Autodesk Inventor part; units mm, degrees
ref_plane "YZ Plane" through (0, 0, 0) normal (1, 0, 0) x (0, 1, 0)
ref_plane "XZ Plane" through (0, 0, 0) normal (0, 1, 0) x (-1, 0, 0)
ref_plane "XY Plane" through (0, 0, 0) normal (0, 0, 1) x (1, 0, 0)
sketch "Sketch1" plane through (0, 0, 0) normal (0, 0, 1) x (1, 0, 0)
  line L0 (0, 0) -> (50.8, 0)
  line L1 (50.8, 0) -> (50.8, 25.4)
  line L2 (50.8, 25.4) -> (0, 25.4)
  line L3 (0, 25.4) -> (0, 0)
  line L4 (3.175, 22.225) -> (47.625, 22.225)
  line L5 (47.625, 22.225) -> (47.625, 3.175)
  line L6 (47.625, 3.175) -> (3.175, 3.175)
  line L7 (3.175, 3.175) -> (3.175, 22.225)
  dimension "d0" = 50.8
  dimension "d1" = 25.4
  dimension "d2" = 3.175
extrude "Extrusion1" add sketch "Sketch1" along normal blind 254
sketch "Sketch2" plane through (0, 0, 0) normal (0, -1, 0) x (1, 0, 0)
  circle A0 centre (25.4, 228.6) radius 4.7625
  line L0 (47.625, 254) -> (3.175, 254)
  line L1 (0, 0) -> (0, 254)
  dimension "d5" = 9.525
  dimension "d6" = 25.4
  dimension "d7" = 25.4
extrude "Extrusion2" cut sketch "Sketch2" against normal blind 25.4
sketch "Sketch3" plane through (0, 25.4, 0) normal (0, 1, 0) x (1, 0, 0)
  circle A0 centre (25.4, -228.6) radius 4.7625
  circle A1 centre (25.4, -228.6) radius 14.2875
  point P0 (0, 0)
  dimension "d10" = 28.575
extrude "Extrusion3" cut sketch "Sketch3" against normal blind 25.4
ref_plane "Work Plane1" through (25.4, 0, 228.6) normal (0, 0, -1) x (1, 0, 0)
sketch "Sketch5" plane through (50.8, 0, 0) normal (1, 0, 0) x (0, 0, -1)
  line L0 (-254, 0) -> (-254, 25.4)
  line L1 (0, 0) -> (-254, 0)
  line L2 (0, 25.4) -> (-254, 25.4)
  point P0 (-215.9, 12.7)
  point P1 (-190.5, 12.7)
  point P2 (-165.1, 12.7)
  point P3 (-241.3, 12.7)
  point P4 (-139.7, 12.7)
  dimension "d21" = 38.1
  dimension "d22" = 12.7
  dimension "d23" = 25.4
  dimension "d24" = 25.4
  dimension "d25" = 12.7
  dimension "d26" = 12.7
  dimension "d57" = 25.4
  dimension "d58" = 25.4
  dimension "d59" = 12.7
  dimension "d60" = 12.7
hole "Hole1" at (50.8, 12.7, 215.9) at (50.8, 12.7, 190.5) at (50.8, 12.7, 165.1) at (50.8, 12.7, 139.7) at (50.8, 12.7, 241.3) direction (-1, 0, 0) diameter 6.7469 end through all
sketch "Sketch6" plane through (0, 25.4, 0) normal (0, 1, 0) x (1, 0, 0)
  line L0 (50.8, 0) -> (50.8, -254)
  line L1 (0, 0) -> (0, -254)
  line L2 (50.8, 0) -> (0, 0)
  point P0 (25.4, -83.3438)
  point P1 (41.275, -25.4)
  point P2 (9.525, -25.4)
  dimension "d42" = 83.3438
  dimension "d43" = 25.4
  dimension "d53" = 57.9438
  dimension "d54" = 57.9438
  dimension "d55" = 15.875
  dimension "d56" = 31.75
hole "Hole2" at (25.4, 25.4, 83.3438) at (41.275, 25.4, 25.4) at (9.525, 25.4, 25.4) direction (0, -1, 0) diameter 5.1594 end through all
properties part number "15102898-16-A-0201" material "Aluminum 6061"
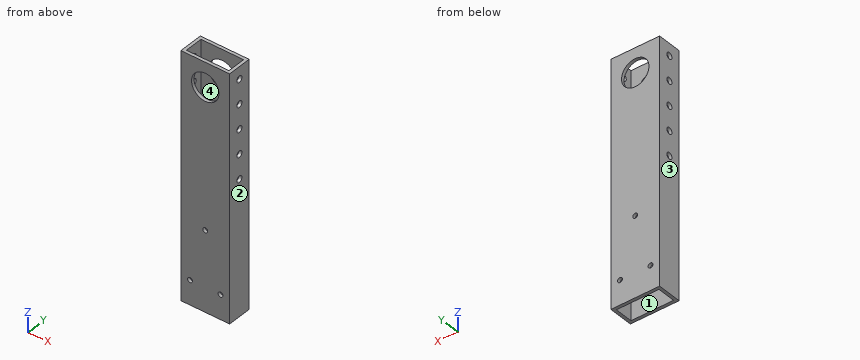
Could you check a few things on this model? Use its own coordinates, in mm. Face numbers are marked on the shaded views. Coordinates: 2 decimals unless noted, no trailing zeros. Loops run counter-clockwise (first coordinate to the right, second up) from the corner with the lowest first, then second, coordinate; pieces in that order, holes last. Notation, with made-up numbers: M 8.5,45.25 L 16.5,45.25 A19 ccw 16.5,65.25 Z; hole C -3,88.5 d4. An arc over 180 degrees is marked long. Put each result on its own line as item: value. Start each with the question number.
(1) Suppose I cut it at C-C on x = 25.4. Please give me the cut outline in (y, z) (1 decimal).
(2) I need wall thicknesses on line 1 (Z direction, x = 25.4, y = 1.4); line 2 (X direction, y = 2.45, z = 25.4); line 3 (X direction, y = 10.25, z = 200.5) (3 decimals). Which ranges of each line are inside material? Lowest first, please. Write a range as from..to.
(3) Suppose I cut it at D-D on z = 32. Please give me the cut outline in (x, y) (3 decimals), then the cut area to 3 significant figures.
(4) Suppose I cut it at B-B on y = 20. Please give me the cut outline in (x, z) (3 decimals).
(5) Thinking about a two-plate mould opening in X: for the marked faces 1, 2, 3 and 4, which applies, pulls with the +X half, pulls with the -X half, needs draft (parallel to the pull), parting line crosses it, or undercut?
(6) Suppose I cut it at A-A on z = 228.6. Please give me the cut outline in (x, y) (1 decimal).
Solutions:
1. outline: M 0,0 L 3.2,0 L 3.2,80.8 L 0,80.8 Z; M 0,85.9 L 3.2,85.9 L 3.2,214.3 L 0,214.3 Z; M 0,242.9 L 3.2,242.9 L 3.2,254 L 0,254 Z; M 22.2,0 L 25.4,0 L 25.4,80.8 L 22.2,80.8 Z; M 22.2,85.9 L 25.4,85.9 L 25.4,214.3 L 22.2,214.3 Z; M 22.2,242.9 L 25.4,242.9 L 25.4,254 L 22.2,254 Z
2. line 1: z = 0..80.76, 85.92..214.31, 242.89..254
2. line 2: x = 0..6.95, 12.1..38.7, 43.85..50.8
2. line 3: x = 0..3.175, 47.625..50.8
3. outline: M 0,0 L 50.8,0 L 50.8,25.4 L 0,25.4 Z; hole M 3.175,3.175 L 47.625,3.175 L 47.625,22.225 L 3.175,22.225 Z
3. area: 444 mm2
4. outline: M 0,0 L 3.175,0 L 3.175,254 L 0,254 Z; M 47.625,0 L 50.8,0 L 50.8,254 L 47.625,254 Z
5. face 1: undercut
5. face 2: pulls with the +X half
5. face 3: pulls with the -X half
5. face 4: undercut
6. outline: M 0,0 L 11.1,0 L 11.1,3.2 L 3.2,3.2 L 3.2,22.2 L 11.1,22.2 L 11.1,25.4 L 0,25.4 Z; M 39.7,0 L 50.8,0 L 50.8,25.4 L 39.7,25.4 L 39.7,22.2 L 47.6,22.2 L 47.6,3.2 L 39.7,3.2 Z
